```python
from build123d import *

# Parameters (mm, degrees)
BOSS_EXTRUDE1_DEPTH     = 11
SKETCH2_W               = 37
SKETCH2_H               = 20
BOSS_EXTRUDE2_DEPTH     = 6
SKETCH8_R               = 8
BOSS_EXTRUDE3_DEPTH     = 5
CUT_EXTRUDE1_DEPTH      = 24.732888573
CUT_EXTRUDE1_DEPTH_BACK = 3
SKETCH4_R               = 4.875
SKETCH5_R               = 2.625
CUT_EXTRUDE2_DEPTH      = 24.732888573
CUT_EXTRUDE3_DEPTH      = 6
SKETCH7_R               = 4.5
CUT_EXTRUDE4_DEPTH      = 24.286262044
FILLET2_R               = 10


with BuildPart() as part:
    # Sketch1 → Boss-Extrude1 (new body)
    with BuildSketch(Plane(origin=(0, 0, 0), x_dir=(1, 0, 0), z_dir=(0, 1, 0))):
        with BuildLine():
            Line((-5, -10), (5, -10))
            ThreePointArc((5, -10), (8.535533906, -8.535533906), (10, -5))
            Line((10, -5), (10, 5))
            ThreePointArc((10, 5), (8.535533906, 8.535533906), (5, 10))
            Line((5, 10), (-5, 10))
            ThreePointArc((-5, 10), (-8.535533906, 8.535533906), (-10, 5))
            Line((-10, 5), (-10, -5))
            ThreePointArc((-10, -5), (-8.535533906, -8.535533906), (-5, -10))
        make_face()
    extrude(amount=-BOSS_EXTRUDE1_DEPTH)

    # Sketch2 → Boss-Extrude2 (add)
    with BuildSketch(Plane(origin=(0, 0, 0), x_dir=(1, 0, 0), z_dir=(0, 1, 0))):
        Rectangle(SKETCH2_W, SKETCH2_H)
    extrude(amount=-BOSS_EXTRUDE2_DEPTH)

    # Sketch8 → Boss-Extrude3 (add)
    with BuildSketch(Plane(origin=(0, 0, 0), x_dir=(1, 0, 0), z_dir=(0, 1, 0))):
        with Locations(Location((0, 0, 0), (0, 0, 90))):
            Circle(SKETCH8_R)
    extrude(amount=BOSS_EXTRUDE3_DEPTH)

    # Sketch4 → Cut-Extrude1 (cut, two sides: drawn at the far end of the back side and taken through both)
    with BuildSketch(Plane(origin=(0, -6, 0), x_dir=(-1, 0, 0), z_dir=(0, -1, 0)).offset(-CUT_EXTRUDE1_DEPTH_BACK)):
        with Locations(Location((-12.7, 0, 0), (0, 0, 303.631277448))):
            Circle(SKETCH4_R)
        with Locations(Location((12.7, 0, 0), (0, 0, 270))):
            Circle(SKETCH4_R)
    extrude(amount=CUT_EXTRUDE1_DEPTH + CUT_EXTRUDE1_DEPTH_BACK, mode=Mode.SUBTRACT)

    # Sketch5 → Cut-Extrude2 (cut, through all)
    with BuildSketch(Plane(origin=(0, -6, 0), x_dir=(-1, 0, 0), z_dir=(0, -1, 0))):
        with Locations(Location((-12.7, 0, 0), (0, 0, 90))):
            Circle(SKETCH5_R)
        with Locations(Location((12.7, 0, 0), (0, 0, 90))):
            Circle(SKETCH5_R)
    extrude(amount=-CUT_EXTRUDE2_DEPTH, mode=Mode.SUBTRACT)

    # Sketch6 → Cut-Extrude3 (cut)
    with BuildSketch(Plane.XZ.offset(11)):
        Polygon((7, -4.041451884), (7, 4.041451884), (0, 8.082903769), (-7, 4.041451884), (-7, -4.041451884), (0, -8.082903769), align=None)
    extrude(amount=-CUT_EXTRUDE3_DEPTH, mode=Mode.SUBTRACT)

    # Sketch7 → Cut-Extrude4 (cut, through all)
    with BuildSketch(Plane.XZ.offset(5)):
        with Locations(Location((0, 0, 0), (0, 0, 270))):
            Circle(SKETCH7_R)
    extrude(amount=-CUT_EXTRUDE4_DEPTH, mode=Mode.SUBTRACT)

    # Fillet2
    fillet2_edges = [part.edges().sort_by_distance(p)[0] for p in [
        (-18.5, -3, 10),
        (-18.5, -3, -10),
        (18.5, -3, -10),
        (18.5, -3, 10),
    ]]
    fillet(fillet2_edges, radius=FILLET2_R - 0.0001)  # a hair under: the kernel refuses the full size


solid = part.part
```
Verification items for the finished model (mm, model axes). A direction names the side the tool comes from. Give positions to 0.01 mm unless a question says otherwise; leave off trailing zeros. Loops run counter-clockwise (first coordinate to the right, second up) from the corner with the lowest first, then second, coordinate; pieces in that order, holes last.
1. Thickness scan on line 1 (X direction, y = -1.15, z = 0) (3 decimals); line 2 (X direction, y = -5.5, z = 0) (3 decimals); line 3 (X direction, y = -6.25, z = 0) (3 decimals). Record the ranges inside material, lowest first.
2. Section check D-D, the plane z = -7.5. Enter the section's corners in (x, y).
3. Section check A-A, the plane x = -12. Enter the section's corners in (y, z).
4. Section check C-C, the plane z = 0.5. Count the separate pieces of the cut face and the enclosed holes in it, then the cut area to 3 significant figures.
5. Set-up check for faces 5 (the flat face through (10, -8.5, 4.5)), 6 (the cylindrical face through (-9, -8, 8)), 7 (the flat face through (-3.2, -5, -3.5)): record each of +Z, -Z, +X, -X, +Y, -Y from which the full face is reachable in a straight line by a thin tool's end or side.
6. Mould release check, pull along Z, two halves, no side actions. Record for faces 1 (the flat face through (-10, -8.5, -4.5)), 2 (the flat face through (0, -4, 10)), 3 (the flat face through (-10.6, -3, 2.1)), 4 (the flat face through (-3.549, -8.042, -6.034)): released by +Z, released by -Z, zero draft, split by the parting line, or undercut.
7. Go/stop test with flat-tipped pins: pin 1 Ø0.8 at (y, z) = (-9.5, -4.5) entering from -X; pin 2 Ø1 at (y, z) = (-5.5, 6.5) entering from -X; pin 3 Ø2 at (y, z) = (-8.5, -7.5) entering from -X; pin 4 Ø8 at (x, z) = (0, 0) entering from -Y. Record where each tip stops, or that it passes through.
8. Section check B-B, the plane y = 2. Enter the section's corners in (x, z).
Geometry says:
1. line 1: x = -18.5 to -15.325, -10.075 to -4.5, 4.5 to 10.075, 15.325 to 18.5
1. line 2: x = -18.5 to -17.575, -7.825 to -7, 7 to 7.825, 17.575 to 18.5
1. line 3: x = -7.825 to -7, 7 to 7.825
2. outline: (-15.11, -6) - (-9.33, -6) - (-9.33, -11) - (-1.01, -11) - (-1.01, -5) - (1.01, -5) - (1.01, -11) - (9.33, -11) - (9.33, -6) - (15.11, -6) - (15.11, 0) - (2.78, 0) - (2.78, 5) - (-2.78, 5) - (-2.78, 0) - (-15.11, 0) - close
3. outline: (-6, -9.37) - (0, -9.37) - (0, -2.53) - (-3, -2.53) - (-3, -4.82) - (-6, -4.82) - close; (-6, 4.82) - (-3, 4.82) - (-3, 2.53) - (0, 2.53) - (0, 9.37) - (-6, 9.37) - close
4. separate pieces: 4
4. enclosed holes: 0
4. area: 118 mm2
5. face 5: +Z, -Z, +X, -Y
5. face 6: +Z, -X, -Y
5. face 7: -Y
6. face 1: zero draft
6. face 2: released by +Z
6. face 3: undercut
6. face 4: undercut
7. pin 1: stops at x = -10
7. pin 2: stops at x = -16.5
7. pin 3: stops at x = -9.77
7. pin 4: passes through
8. outline: circle Ø16 at (0, 0); hole circle Ø9 at (0, 0)
